Read the model definition and answer for the solid it produces. Units are mm, in the model's axes. Face numbers are marked on the shaded views. A direction names the side the tool comes from. Round coordinates to 2 decimals unless told otherwise and drop trailing zeros. Order: outer loops, then holes, each group sorted by start corner. A loop starts at its lowest first (then second) coordinate and runs counter-clockwise, first axis right, second up.
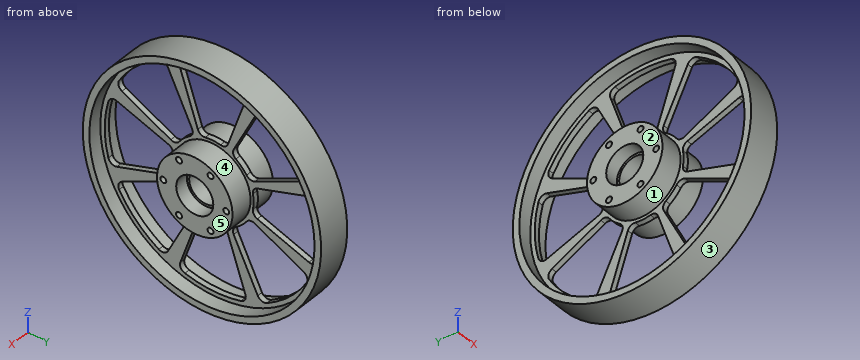
from build123d import *

# Parameters (mm, degrees)
SKETCH2_R          = 2.25
CUT_EXTRUDE1_DEPTH = 40
CUT_EXTRUDE2_DEPTH = 40


with BuildPart() as part:
    # Sketch1 → Revolve1 (revolve)
    with BuildSketch(Plane(origin=(0, 0, 0), x_dir=(1, 0, 0), z_dir=(0, 1, 0)), mode=Mode.PRIVATE) as revolve1_sk:
        Polygon((-9, 12.25), (9, 12.25), (9, 14), (19, 14), (19, 28.5), (2, 28.5), (2, 85), (12.25, 85), (12.25, 90), (-12.25, 90), (-12.25, 85), (-2, 85), (-2, 28.5), (-19, 28.5), (-19, 14), (-9, 14), align=None)
    revolve(revolve1_sk.sketch.rotate(Axis((0, 0, 0), (1, 0, 0)), 180), axis=Axis((0, 0, 0), (1, 0, 0)))

    # Sketch2 → Cut-Extrude1 (cut)
    with BuildSketch(Plane(origin=(19, 0, 0), x_dir=(0, 0, -1), z_dir=(1, 0, 0))):
        with Locations((0, 23.75)):
            Circle(SKETCH2_R)
        with Locations((20.56810334, 11.875)):
            Circle(SKETCH2_R)
        with Locations((20.56810334, -11.875)):
            Circle(SKETCH2_R)
        with Locations((0, -23.75)):
            Circle(SKETCH2_R)
        with Locations((-20.56810334, -11.875)):
            Circle(SKETCH2_R)
        with Locations((-20.56810334, 11.875)):
            Circle(SKETCH2_R)
    extrude(amount=-CUT_EXTRUDE1_DEPTH, mode=Mode.SUBTRACT)

    # Sketch3 → Cut-Extrude2 (cut)
    with BuildSketch(Plane.ZY.offset(2)):
        with BuildLine():
            Line((33.864614623, 68.618602963), (15.68286139, 31.777595908))
            ThreePointArc((15.68286139, 31.777595908), (15.330601224, 28.294565139), (17.34904213, 25.434235286))
            ThreePointArc((17.34904213, 25.434235286), (21.770273165, 21.770273165), (25.434235286, 17.34904213))
            ThreePointArc((25.434235286, 17.34904213), (28.294565139, 15.330601224), (31.777595908, 15.68286139))
            Line((31.777595908, 15.68286139), (68.618602963, 33.864614623))
            ThreePointArc((68.618602963, 33.864614623), (71.190803513, 36.897849656), (70.735686396, 40.848748142))
            ThreePointArc((70.735686396, 40.848748142), (57.758798268, 57.758798268), (40.848748142, 70.735686396))
            ThreePointArc((40.848748142, 70.735686396), (36.897849656, 71.190803513), (33.864614623, 68.618602963))
        make_face()
        with BuildLine():
            Line((72.466578112, 24.574780828), (33.559611194, 11.380695919))
            ThreePointArc((33.559611194, 11.380695919), (30.847650966, 9.166906795), (30.252345582, 5.717094908))
            ThreePointArc((30.252345582, 5.717094908), (30.787815567, 0), (30.252345582, -5.717094908))
            ThreePointArc((30.252345582, -5.717094908), (30.847650966, -9.166906795), (33.559611194, -11.380695919))
            Line((33.559611194, -11.380695919), (72.466578112, -24.574780828))
            ThreePointArc((72.466578112, -24.574780828), (76.430219625, -24.248780219), (78.902110336, -21.133256708))
            ThreePointArc((78.902110336, -21.133256708), (81.683275856, 0), (78.902110336, 21.133256708))
            ThreePointArc((78.902110336, 21.133256708), (76.430219625, 24.248780219), (72.466578112, 24.574780828))
        make_face()
        with BuildLine():
            Line((-24.574780828, 72.466578112), (-11.380695919, 33.559611194))
            ThreePointArc((-11.380695919, 33.559611194), (-9.166906795, 30.847650966), (-5.717094908, 30.252345582))
            ThreePointArc((-5.717094908, 30.252345582), (0, 30.787815567), (5.717094908, 30.252345582))
            ThreePointArc((5.717094908, 30.252345582), (9.166906795, 30.847650966), (11.380695919, 33.559611194))
            Line((11.380695919, 33.559611194), (24.574780828, 72.466578112))
            ThreePointArc((24.574780828, 72.466578112), (24.248780219, 76.430219625), (21.133256708, 78.902110336))
            ThreePointArc((21.133256708, 78.902110336), (0, 81.683275856), (-21.133256708, 78.902110336))
            ThreePointArc((-21.133256708, 78.902110336), (-24.248780219, 76.430219625), (-24.574780828, 72.466578112))
        make_face()
        with BuildLine():
            Line((68.618602963, -33.864614623), (31.777595908, -15.68286139))
            ThreePointArc((31.777595908, -15.68286139), (28.294565139, -15.330601224), (25.434235286, -17.34904213))
            ThreePointArc((25.434235286, -17.34904213), (21.770273165, -21.770273165), (17.34904213, -25.434235286))
            ThreePointArc((17.34904213, -25.434235286), (15.330601224, -28.294565139), (15.68286139, -31.777595908))
            Line((15.68286139, -31.777595908), (33.864614623, -68.618602963))
            ThreePointArc((33.864614623, -68.618602963), (36.897849656, -71.190803513), (40.848748142, -70.735686396))
            ThreePointArc((40.848748142, -70.735686396), (57.758798268, -57.758798268), (70.735686396, -40.848748142))
            ThreePointArc((70.735686396, -40.848748142), (71.190803513, -36.897849656), (68.618602963, -33.864614623))
        make_face()
        with BuildLine():
            Line((24.574780828, -72.466578112), (11.380695919, -33.559611194))
            ThreePointArc((11.380695919, -33.559611194), (9.166906795, -30.847650966), (5.717094908, -30.252345582))
            ThreePointArc((5.717094908, -30.252345582), (0, -30.787815567), (-5.717094908, -30.252345582))
            ThreePointArc((-5.717094908, -30.252345582), (-9.166906795, -30.847650966), (-11.380695919, -33.559611194))
            Line((-11.380695919, -33.559611194), (-24.574780828, -72.466578112))
            ThreePointArc((-24.574780828, -72.466578112), (-24.248780219, -76.430219625), (-21.133256708, -78.902110336))
            ThreePointArc((-21.133256708, -78.902110336), (0, -81.683275856), (21.133256708, -78.902110336))
            ThreePointArc((21.133256708, -78.902110336), (24.248780219, -76.430219625), (24.574780828, -72.466578112))
        make_face()
        with BuildLine():
            Line((-33.864614623, -68.618602963), (-15.68286139, -31.777595908))
            ThreePointArc((-15.68286139, -31.777595908), (-15.330601224, -28.294565139), (-17.34904213, -25.434235286))
            ThreePointArc((-17.34904213, -25.434235286), (-21.770273165, -21.770273165), (-25.434235286, -17.34904213))
            ThreePointArc((-25.434235286, -17.34904213), (-28.294565139, -15.330601224), (-31.777595908, -15.68286139))
            Line((-31.777595908, -15.68286139), (-68.618602963, -33.864614623))
            ThreePointArc((-68.618602963, -33.864614623), (-71.190803513, -36.897849656), (-70.735686396, -40.848748142))
            ThreePointArc((-70.735686396, -40.848748142), (-57.758798268, -57.758798268), (-40.848748142, -70.735686396))
            ThreePointArc((-40.848748142, -70.735686396), (-36.897849656, -71.190803513), (-33.864614623, -68.618602963))
        make_face()
        with BuildLine():
            Line((-72.466578112, -24.574780828), (-33.559611194, -11.380695919))
            ThreePointArc((-33.559611194, -11.380695919), (-30.847650966, -9.166906795), (-30.252345582, -5.717094908))
            ThreePointArc((-30.252345582, -5.717094908), (-30.787815567, 0), (-30.252345582, 5.717094908))
            ThreePointArc((-30.252345582, 5.717094908), (-30.847650966, 9.166906795), (-33.559611194, 11.380695919))
            Line((-33.559611194, 11.380695919), (-72.466578112, 24.574780828))
            ThreePointArc((-72.466578112, 24.574780828), (-76.430219625, 24.248780219), (-78.902110336, 21.133256708))
            ThreePointArc((-78.902110336, 21.133256708), (-81.683275856, 0), (-78.902110336, -21.133256708))
            ThreePointArc((-78.902110336, -21.133256708), (-76.430219625, -24.248780219), (-72.466578112, -24.574780828))
        make_face()
        with BuildLine():
            Line((-68.618602963, 33.864614623), (-31.777595908, 15.68286139))
            ThreePointArc((-31.777595908, 15.68286139), (-28.294565139, 15.330601224), (-25.434235286, 17.34904213))
            ThreePointArc((-25.434235286, 17.34904213), (-21.770273165, 21.770273165), (-17.34904213, 25.434235286))
            ThreePointArc((-17.34904213, 25.434235286), (-15.330601224, 28.294565139), (-15.68286139, 31.777595908))
            Line((-15.68286139, 31.777595908), (-33.864614623, 68.618602963))
            ThreePointArc((-33.864614623, 68.618602963), (-36.897849656, 71.190803513), (-40.848748142, 70.735686396))
            ThreePointArc((-40.848748142, 70.735686396), (-57.758798268, 57.758798268), (-70.735686396, 40.848748142))
            ThreePointArc((-70.735686396, 40.848748142), (-71.190803513, 36.897849656), (-68.618602963, 33.864614623))
        make_face()
    extrude(amount=-CUT_EXTRUDE2_DEPTH, mode=Mode.SUBTRACT)


solid = part.part
Q1. Straight lines are drawn through the part: probe 1 along Y at (x, z) = (-9.5, 0); probe 2 along Y at (x, z) = (14.5, 0); probe 3 along Z at (x, y) = (9.5, -1). For each, find the intervals that lie inside material, in ascending order.
Outcome:
probe 1: y = -90 to -85, -28.5 to -26, -21.5 to -14, 14 to 21.5, 26 to 28.5, 85 to 90
probe 2: y = -28.5 to -26, -21.5 to -14, 14 to 21.5, 26 to 28.5
probe 3: z = -89.99 to -84.99, -28.48 to -13.96, 13.96 to 28.48, 84.99 to 89.99
Q2. For a pull along Y with two mould halves and no side action, classify the marked faces 1, 2 and 3 as released by +Y, released by -Y, zero draft, split by the parting line, or undercut.
Outcome:
face 1: undercut
face 2: zero draft
face 3: split by the parting line
Q3. For the marked faces 4 and 5, determine the directions among +Z, -Z, +X, -X, +Y, -Y from which every point of the face is accessible in a straight line to the end or side of a thin tool.
Outcome:
face 4: +X
face 5: +Z, -Z, +X, +Y, -Y
Q4. A cutting plane is placed at B-B, the plane y = -61. Give the vertices of the cut face in (x, z), plus the area to 3 significant figures.
Outcome:
outline: (-12.25, -66.17) - (12.25, -66.17) - (12.25, -59.19) - (2, -59.19) - (2, -54.32) - (-2, -54.32) - (-2, -59.19) - (-12.25, -59.19) - close; (-12.25, 59.19) - (-2, 59.19) - (-2, 54.32) - (2, 54.32) - (2, 59.19) - (12.25, 59.19) - (12.25, 66.17) - (-12.25, 66.17) - close; (-2, -30.1) - (2, -30.1) - (2, -20.69) - (-2, -20.69) - close; (-2, 20.69) - (2, 20.69) - (2, 30.1) - (-2, 30.1) - close
area: 456 mm2
Q5. Flat-ended cylindrical pins translate along their axes: pin 1 (6 mm diameter, centred on x = -15, z = 42.5, fed in from -Y); pin 2 (6 mm diameter, centred on y = -26.5, z = 57, fed in from -X); pin 3 (10 mm diameter, centred on x = -10, z = 20, fed in from +Y). Find the tip coordinate at first contact, or state that the pin passes through.
Outcome:
pin 1: stops at y = -79.96
pin 2: stops at x = -2
pin 3: stops at y = 88.74
Q6. A cutting plane is placed at A-A, the plane z = 44. Give the vertices of the cut face in (x, y), plus the area to 3 significant figures.
Outcome:
outline: (-12.25, -78.51) - (12.25, -78.51) - (12.25, -72.73) - (2, -72.73) - (2, -68.82) - (-2, -68.82) - (-2, -72.73) - (-12.25, -72.73) - close; (-12.25, 72.73) - (-2, 72.73) - (-2, 68.82) - (2, 68.82) - (2, 72.73) - (12.25, 72.73) - (12.25, 78.51) - (-12.25, 78.51) - close; (-2, -21.71) - (2, -21.71) - (2, -14.92) - (-2, -14.92) - close; (-2, 14.92) - (2, 14.92) - (2, 21.71) - (-2, 21.71) - close
area: 369 mm2
Q7. A cutting plane is placed at C-C, the plane z = 0. Give the number of separate pieces and of enclosed holes in the cut face, plus the area to 3 significant figures.
Outcome:
separate pieces: 6
enclosed holes: 0
area: 1,110 mm2
